Input: part model. Units: mm. Frame: model coordinates. Round coordinates to 2 decimals unless told otherwise and drop trailing zeros. Order: outer loops, then holes, each group sorted by start corner. A loop starts at its lowest first (then second) coordinate and runs counter-clockwise, first axis right, second up. Notation, with made-up numbers: (49.5, 29.5) -> (66.5, 29.5) arc R19 cw to (66.5, 64.5) -> close; hole circle Ø11 at (23, 38). An arc over 180 degrees is marked (long way). Answer as CSV lines item,"result". Start each with the question number.
1) Section query C-C, the plane y = 22.5. Output: boundary loops of the cut face in (x, z).
2) Mould query, pull axis X, two halves, no side actions, for faces 1 (the face through (0, 25, 1)), 2 (the face through (12, 0, 0)), 3 (the face through (-5.799, -26.114, 0.986)). Classes: +X half, -X half, draft (parallel to the pull), parting line (faces both ways), or undercut.
3) Line query: L1, parallel to Y at x = 21.5, z = 0.2; L2, parallel to Y at x = -5, z = 0.4; L3, parallel to Y at x = -10.5, z = 1.75. Output: solid intervals per line, ascending.
4) Section query A-A, the plane x = 0. Output: boundary loops of the cut face in (y, z).
5) Section query D-D, the plane z = 1. State how many separate pieces and enclosed holes the cut face has, and give its area (3 significant figures).
6) Section query B-B, the plane x = 11. Output: boundary loops of the cut face in (y, z), and give its area (3 significant figures).
```python
from build123d import *

# Parameters (mm, degrees)
SKETCH1_R           = 26.75
SKETCH1_R_2         = 10
SKETCH1_R_3         = 2.5
SKETCH1_R_4         = 3
BOSS_EXTRUDE1_DEPTH = 2


with BuildPart() as part:
    # Sketch1 → Boss-Extrude1 (new body)
    with BuildSketch(Plane.XY):
        Circle(SKETCH1_R)
        Circle(SKETCH1_R_2, mode=Mode.SUBTRACT)
        with Locations((0, 22.5)):
            Circle(SKETCH1_R_3, mode=Mode.SUBTRACT)
        with Locations((7.695453225, 21.143083968)):
            Circle(SKETCH1_R_3, mode=Mode.SUBTRACT)
        with Locations((14.462721218, 17.23599997)):
            Circle(SKETCH1_R_3, mode=Mode.SUBTRACT)
        with Locations((19.485571585, 11.25)):
            Circle(SKETCH1_R_3, mode=Mode.SUBTRACT)
        with Locations((22.158174443, 3.907083998)):
            Circle(SKETCH1_R_3, mode=Mode.SUBTRACT)
        with Locations((22.158174443, -3.907083998)):
            Circle(SKETCH1_R_3, mode=Mode.SUBTRACT)
        with Locations((19.485571585, -11.25)):
            Circle(SKETCH1_R_3, mode=Mode.SUBTRACT)
        with Locations((14.462721218, -17.23599997)):
            Circle(SKETCH1_R_3, mode=Mode.SUBTRACT)
        with Locations((7.695453225, -21.143083968)):
            Circle(SKETCH1_R_3, mode=Mode.SUBTRACT)
        with Locations((0, -22.5)):
            Circle(SKETCH1_R_3, mode=Mode.SUBTRACT)
        with Locations((-7.695453225, -21.143083968)):
            Circle(SKETCH1_R_3, mode=Mode.SUBTRACT)
        with Locations((-14.462721218, -17.23599997)):
            Circle(SKETCH1_R_3, mode=Mode.SUBTRACT)
        with Locations((-19.485571585, -11.25)):
            Circle(SKETCH1_R_3, mode=Mode.SUBTRACT)
        with Locations((-22.158174443, -3.907083998)):
            Circle(SKETCH1_R_3, mode=Mode.SUBTRACT)
        with Locations((-22.158174443, 3.907083998)):
            Circle(SKETCH1_R_3, mode=Mode.SUBTRACT)
        with Locations((-19.485571585, 11.25)):
            Circle(SKETCH1_R_3, mode=Mode.SUBTRACT)
        with Locations((-14.462721218, 17.23599997)):
            Circle(SKETCH1_R_3, mode=Mode.SUBTRACT)
        with Locations((-7.695453225, 21.143083968)):
            Circle(SKETCH1_R_3, mode=Mode.SUBTRACT)
        with Locations((0, 15)):
            Circle(SKETCH1_R_4, mode=Mode.SUBTRACT)
        with Locations((9.641814145, 11.490666647)):
            Circle(SKETCH1_R_4, mode=Mode.SUBTRACT)
        with Locations((14.772116295, 2.604722665)):
            Circle(SKETCH1_R_4, mode=Mode.SUBTRACT)
        with Locations((12.990381057, -7.5)):
            Circle(SKETCH1_R_4, mode=Mode.SUBTRACT)
        with Locations((5.13030215, -14.095389312)):
            Circle(SKETCH1_R_4, mode=Mode.SUBTRACT)
        with Locations((-5.13030215, -14.095389312)):
            Circle(SKETCH1_R_4, mode=Mode.SUBTRACT)
        with Locations((-12.990381057, -7.5)):
            Circle(SKETCH1_R_4, mode=Mode.SUBTRACT)
        with Locations((-14.772116295, 2.604722665)):
            Circle(SKETCH1_R_4, mode=Mode.SUBTRACT)
        with Locations((-9.641814145, 11.490666647)):
            Circle(SKETCH1_R_4, mode=Mode.SUBTRACT)
    extrude(amount=BOSS_EXTRUDE1_DEPTH)


solid = part.part
```
Findings:
1,outline,"(-14.47, 0) -> (-9.8, 0) -> (-9.8, 2) -> (-14.47, 2) -> close; (-5.6, 0) -> (-2.5, 0) -> (-2.5, 2) -> (-5.6, 2) -> close; (2.5, 0) -> (5.6, 0) -> (5.6, 2) -> (2.5, 2) -> close; (9.8, 0) -> (14.47, 0) -> (14.47, 2) -> (9.8, 2) -> close"
2,face 1,"undercut"
2,face 2,"draft"
2,face 3,"parting line"
3,L1,"y = -15.92 to -12.73, -9.77 to -6.32, -1.5 to 1.5, 6.32 to 9.77, 12.73 to 15.92"
3,L2,"y = -26.28 to -17.09, -11.1 to -8.66, 8.66 to 26.28"
3,L3,"y = -24.6 to -9.17, -5.83 to 8.62, 14.37 to 24.6"
4,outline,"(-26.75, 0) -> (-25, 0) -> (-25, 2) -> (-26.75, 2) -> close; (-20, 0) -> (-10, 0) -> (-10, 2) -> (-20, 2) -> close; (10, 0) -> (12, 0) -> (12, 2) -> (10, 2) -> close; (18, 0) -> (20, 0) -> (20, 2) -> (18, 2) -> close; (25, 0) -> (26.75, 0) -> (26.75, 2) -> (25, 2) -> close"
5,separate pieces,"1"
5,enclosed holes,"28"
5,area,"1,330 mm^2"
6,outline,"(-24.38, 0) -> (-9.74, 0) -> (-9.74, 2) -> (-24.38, 2) -> close; (-5.26, 0) -> (8.82, 0) -> (8.82, 2) -> (-5.26, 2) -> close; (14.17, 0) -> (24.38, 0) -> (24.38, 2) -> (14.17, 2) -> close"
6,area,"77.9 mm^2"
